```python
from build123d import *

# Parameters (mm, degrees)
SKETCH1_W           = 171
SKETCH1_H           = 70
SKETCH1_R           = 2.25
BOSS_EXTRUDE1_DEPTH = 5
SKETCH2_W           = 171
SKETCH2_H           = 65
SKETCH2_R           = 2.25
BOSS_EXTRUDE2_DEPTH = 3
CHAMFER1_SIZE       = 8
CHAMFER3_SIZE       = 3
SKETCH3_W           = 7.071067812
SKETCH3_H           = 2.6
CUT_EXTRUDE1_DEPTH  = 199.002168661
SKETCH4_R           = 29
SKETCH4_R_2         = 1.75
CUT_EXTRUDE2_DEPTH  = 185.945938047


with BuildPart() as part:
    # Sketch1 → Boss-Extrude1 (new body)
    with BuildSketch(Plane.XY):
        with Locations((85.5, 35)):
            Rectangle(SKETCH1_W, SKETCH1_H)
        with Locations((15, 9)):
            Circle(SKETCH1_R, mode=Mode.SUBTRACT)
        with Locations(Location((156, 9, 0), (0, 0, 180))):
            Circle(SKETCH1_R, mode=Mode.SUBTRACT)
        with Locations((15, 58)):
            Circle(SKETCH1_R, mode=Mode.SUBTRACT)
        with Locations(Location((156, 58, 0), (0, 0, 180))):
            Circle(SKETCH1_R, mode=Mode.SUBTRACT)
    extrude(amount=-BOSS_EXTRUDE1_DEPTH)

    # Sketch2 → Boss-Extrude2 (add)
    with BuildSketch(Plane(origin=(0, 0, -5), x_dir=(-1, 0, 0), z_dir=(0, 0, -1))):
        with Locations((-85.5, 37.5)):
            Rectangle(SKETCH2_W, SKETCH2_H)
        with Locations(Location((-15, 9, 0), (0, 0, 180))):
            Circle(SKETCH2_R, mode=Mode.SUBTRACT)
        with Locations((-156, 9)):
            Circle(SKETCH2_R, mode=Mode.SUBTRACT)
        with Locations(Location((-15, 58, 0), (0, 0, 180))):
            Circle(SKETCH2_R, mode=Mode.SUBTRACT)
        with Locations((-156, 58)):
            Circle(SKETCH2_R, mode=Mode.SUBTRACT)
    extrude(amount=BOSS_EXTRUDE2_DEPTH)

    # Chamfer1
    # the kernel refuses this chamfer: 8 mm, written as the material it takes off along each edge
    with BuildSketch(Plane(origin=(171, -15.573463904, -8), x_dir=(-0.9996219169112968, 0, -0.027495876610586296), z_dir=(0, 1, 0)), Plane(origin=(0, 90.573463904, -8), x_dir=(0.9996219169112968, 0, -0.027495876610586275), z_dir=(0, -1, 0))) as chamfer1_piece_1:
        Polygon((CHAMFER1_SIZE * 0.999621916911, CHAMFER1_SIZE * 0.0274958766106), (-CHAMFER1_SIZE * 0.0274958766106, CHAMFER1_SIZE * 0.999621916911), (0, 0), align=None)
    extrude(amount=106.146927807, mode=Mode.SUBTRACT)

    # Chamfer3
    chamfer3_edges = [part.edges().sort_by_distance(p)[0] for p in [
        (85.5, 70, -8),
    ]]
    chamfer(chamfer3_edges, length=CHAMFER3_SIZE)

    # Sketch3 → Cut-Extrude1 (cut, through all, along a direction that is not the sketch's normal)
    with BuildSketch(Plane(origin=(85.5, 0, -85.5), x_dir=(-0.7071067811865452, 0, -0.7071067811865498), z_dir=(0.7071067811865498, 0, -0.7071067811865452))):
        with Locations((-117.379725677, 1.3)):
            Rectangle(SKETCH3_W, SKETCH3_H)
    extrude(amount=-CUT_EXTRUDE1_DEPTH, dir=(1, 0, 0), mode=Mode.SUBTRACT)

    # Sketch4 → Cut-Extrude2 (cut, through all)
    with BuildSketch(Plane.XY):
        with Locations((58, 36.3)):
            Circle(SKETCH4_R)
        with Locations((33, 60.3)):
            Circle(SKETCH4_R_2)
        with Locations((83, 60.3)):
            Circle(SKETCH4_R_2)
        with Locations((83, 10.3)):
            Circle(SKETCH4_R_2)
        with Locations((33, 10.3)):
            Circle(SKETCH4_R_2)
    extrude(amount=-CUT_EXTRUDE2_DEPTH, mode=Mode.SUBTRACT)


solid = part.part
```
Could you check a few things on this model? Use its own coordinates, in mm. A direction names the side the tool comes from. Coordinates: 2 decimals unless noted, no trailing zeros. Order: outer loops, then holes, each group sorted by start corner. A loop starts at its lowest first (then second) coordinate and runs counter-clockwise, first axis right, second up. Notation, with made-up numbers: M 61.5,4 L 114.5,4 A24 cw 114.5,39 Z; hole C 84,58 d2. An arc over 180 degrees is marked long. Use a Markdown table: item, result. Add a question column.
Q1. We'd pull the mould along Y, two halves only. Please class faces 1 (the flat face through (103, 37, 0)), 2 (the cylindrical face through (84.669, 10.826, -3.944)), 3 (the flat face through (87, 68, -7)): pulls with the +Y half, pulls with the -Y half, needs draft (parallel to the pull), parting line crosses it, or undercut.
Q2. I want a section at C-C on y = 49. List the corners of the cut face in (x, z) for me, then the cut area to 3 significant figures.
Q3. I want a section at A-A on z = -3. Give the number of separate pieces and of enclosed holes in the cut face, then the cut area to 3 significant figures.
Q4. I want a section at D-D on x = 83. List the corners of the cut face in (y, z) for me.
Q5. If I drill on L1, parallel to Y at x = 156, z = -3.5; L2, parallel to Y at x = 15, z = -6.4; L3, parallel to Y at x = 58, z = -4.5, over which ranges is the centre line in solid material (lowest first)?
Q6. I'm going to push flat-ended pins straight in: pin 1 (2 mm diameter, centred on y = 55, z = -2.5, fed in from +X); pin 2 (2 mm diameter, centred on y = 17.5, z = -5, fed in from +X); pin 3 (1.2 mm diameter, centred on x = 90, y = 4, fed in from -Z). Where does each tip first touch, or does it pass through?
Q7. Which directions (+Z, -Z, +X, -X, +Y, -Y) give clear straight access to the entire face, cutting with the end or side of a thin tool? Please do faces 4 (the flat face through (87, 5, -6)), 5 (the cylindrical face through (31.71, 11.48, -3.94)).
Q8. I want a section at B-B on x = 15. List the corners of the cut face in (y, z) for me.
Checked values:
| question | item | result |
|---|---|---|
| 1 | face 1 | needs draft |
| 1 | face 2 | undercut |
| 1 | face 3 | pulls with the +Y half |
| 2 | outline | M 0,0 L 8,-8 L 31.93,-8 L 31.93,0 Z; M 84.07,-8 L 163,-8 L 171,0 L 84.07,0 Z |
| 2 | area | 887 mm² |
| 3 | separate pieces | 1 |
| 3 | enclosed holes | 9 |
| 3 | area | 8,380 mm² |
| 4 | outline | M 2.6,-5 L 5,-5 L 5,-8 L 8.55,-8 L 8.55,0 L 2.6,0 Z; M 12.05,-8 L 21.6,-8 L 21.6,0 L 12.05,0 Z; M 51,-8 L 58.55,-8 L 58.55,0 L 51,0 Z; M 62.05,-8 L 67,-8 L 70,-5 L 70,0 L 62.05,0 Z |
| 5 | L1 | 2.6 to 6.75, 11.25 to 55.75, 60.25 to 70 |
| 5 | L2 | 5 to 6.75, 11.25 to 55.75, 60.25 to 68.6 |
| 5 | L3 | 2.6 to 7.3, 65.3 to 70 |
| 6 | pin 1 | x = 169.5 |
| 6 | pin 2 | x = 167 |
| 6 | pin 3 | z = -5 |
| 7 | face 4 | -Z, +X, -X, -Y |
| 7 | face 5 | +Z, -Z |
| 8 | outline | M 2.6,-5 L 5,-5 L 5,-8 L 6.75,-8 L 6.75,0 L 2.6,0 Z; M 11.25,-8 L 55.75,-8 L 55.75,0 L 11.25,0 Z; M 60.25,-8 L 67,-8 L 70,-5 L 70,0 L 60.25,0 Z |
